Answer from the drawing. Dimensions are ordinates in mm from the lowest x, y and z of the part. Round coordinates to 2 decimals unless told otherwise and drop trailing zeros. Loops run counter-clockwise (first coordinate to the right, second up) from the corner with the lowest first, then second, coordinate; pieces in that order, holes last.
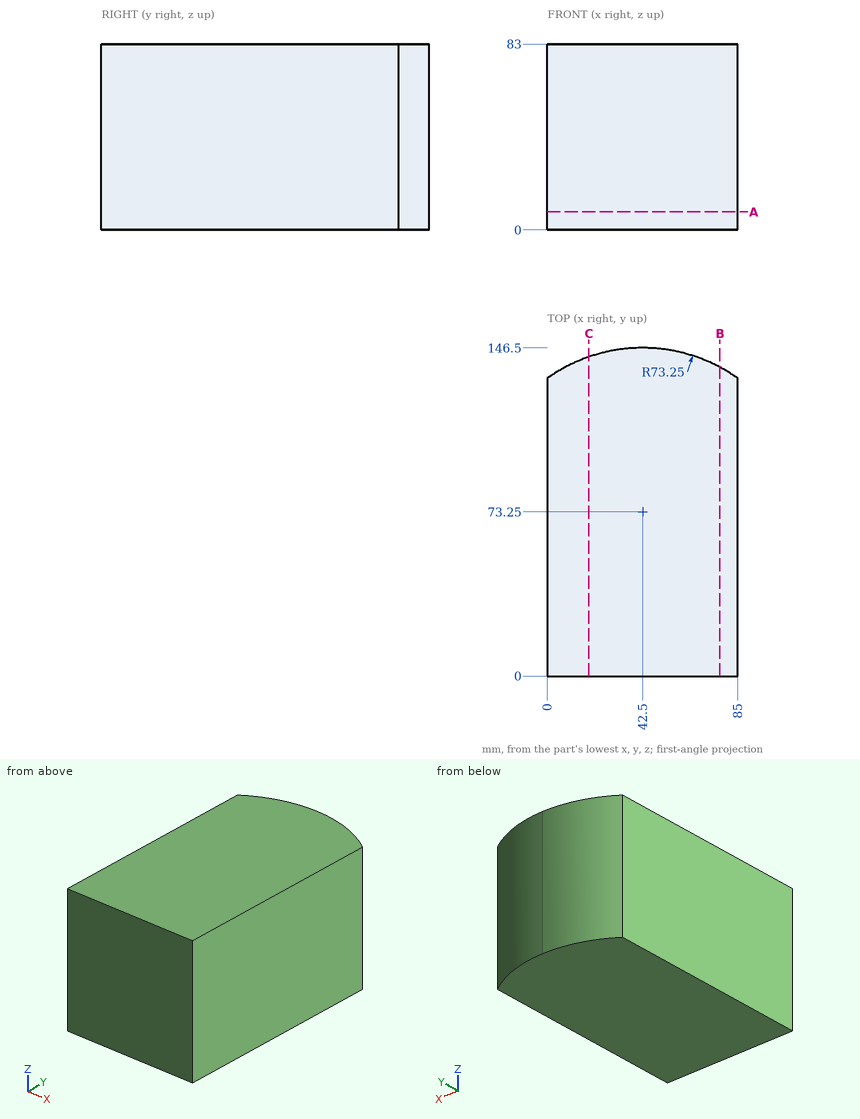
Item 1: Straight lines are drawn through the part: line 1 (Y direction, x = 42, z = 42.5); line 2 (Y direction, x = 71, z = 43.5). For each, find the intervals that lie inside material, in ascending order.
Item 2: Section C-C, the plane x = 18.5 is taken. Give the vertices of the cut face in (y, z).
Item 3: Section A-A, the plane z = 8 is taken. Give the vertices of the cut face in (x, y), plus the area to 3 significant figures.
Item 4: This flat-tipped pin is pushed along its axis until it touches: P1, Ø2, axis at x = 66.5, z = 18.5, coming from the +Y side. Where does it stop, or does it pass through?
Item 5: Section B-B, the plane x = 77 is taken. Give the vertices of the cut face in (y, z).
Answer below:
1. line 1: y = 0 to 146.5
1. line 2: y = 0 to 140.73
2. outline: (0, 0) - (142.46, 0) - (142.46, 83) - (0, 83) - close
3. outline: (0, 0) - (85, 0) - (85, 132.91) arc R73.25 ccw to (0, 132.91) - close
3. area: 12,100 mm2
4. P1: stops at y = 142.8
5. outline: (0, 0) - (137.87, 0) - (137.87, 83) - (0, 83) - close
